Verification items for the finished model (mm, model axes). A direction names the side the tool comes from. Coordinates: 2 decimals unless noted, no trailing zeros. Loops run counter-clockwise (first coordinate to the right, second up) from the corner with the lowest first, then second, coordinate; pieces in that order, holes last. Notation, with made-up numbers: (12.5, -25) - (39.5, -25) arc R20 cw to (39.5, -1) - close; hole circle Ø10 at (-19.75, 0). An arc over 180 degrees is marked (long way). One line per item, written item: value. Start each with the question number.
(1) Set-up check for faces 4 (the face through (111, 69, 3)), 5 (the face through (64, 25, 28)): record each of +Z, -Z, +X, -X, +Y, -Y from which the full face is reachable in a straight line by a thin tool's end or side.
(2) Thickness scan on probe 1 along Y at (x, z) = (16.63, 16.25); probe 2 along Y at (x, z) = (49, 11.5); probe 3 along Y at (x, z) = (63.88, 14.25). Record the ranges inside material, lowest first. Write a range as [from, to].
(3) Draft check along X on faces 1 (the face through (92.562, 10.878, 13.919)), 2 (the face through (64, 4, 28)), 3 (the face through (0, 42, 14)). Enter one of: +X half, -X half, draft (parallel to the pull), parting line (faces both ways), or undercut.
(4) Gauge pin test, flat ends, axial feed: P1, Ø14, axis at x = 82.5, y = 14.5, coming from the +Z side; P2, Ø1.5, axis at x = 27, y = 56, coming from the +Z side; P3, Ø22.5, axis at x = 94, y = 46.5, coming from the +Z side. Record the tip position at first contact, or that the pin passes through.
(5) Section check A-A (z = 13.25). Count the separate pieces of the cut face and the enclosed holes in it, plus the area to 3 significant figures.
(6) Section check B-B (y = 42.74). Record the boundary of the cut face in (x, z), plus the area to 3 significant figures.
```python
from build123d import *

# Parameters (mm, degrees)
ESQUISSE1_W             = 127.76
ESQUISSE1_H             = 85.48
BOSS_EXTRU_1_DEPTH      = 28
ESQUISSE2_R             = 14
ENL_V_MAT_EXTRU_1_DEPTH = 25
CHANFREIN1_SIZE         = 2
CHANFREIN1_SIZE_2       = 3.464101615


with BuildPart() as part:
    # Esquisse1 → Boss.-Extru.1 (new body)
    with BuildSketch(Plane.XY):
        with Locations((63.88, 42.74)):
            Rectangle(ESQUISSE1_W, ESQUISSE1_H)
    extrude(amount=BOSS_EXTRU_1_DEPTH)

    # Esquisse2 → Enlèv. mat.-Extru.1 (cut)
    with BuildSketch(Plane.XY.offset(28)):
        with Locations((111.13, 69.24)):
            Circle(ESQUISSE2_R)
        with Locations((79.63, 69.24)):
            Circle(ESQUISSE2_R)
        with Locations((48.13, 69.24)):
            Circle(ESQUISSE2_R)
        with Locations((16.63, 69.24)):
            Circle(ESQUISSE2_R)
        with Locations((32.38, 42.74)):
            Circle(ESQUISSE2_R)
        with Locations((16.63, 16.24)):
            Circle(ESQUISSE2_R)
        with Locations((48.13, 16.24)):
            Circle(ESQUISSE2_R)
        with Locations((111.13, 16.24)):
            Circle(ESQUISSE2_R)
        with Locations((79.63, 16.24)):
            Circle(ESQUISSE2_R)
        with Locations((63.88, 42.74)):
            Circle(ESQUISSE2_R)
        with Locations((95.38, 42.74)):
            Circle(ESQUISSE2_R)
    extrude(amount=-ENL_V_MAT_EXTRU_1_DEPTH, mode=Mode.SUBTRACT)

    # Chanfrein1
    # the kernel refuses this chamfer: 3.464101615, 2 mm, written as the material it takes off along each edge
    with BuildSketch(Plane(origin=(79.63, 69.24, 28), x_dir=(1, 0, 0), z_dir=(0, -1, 0))) as chanfrein1_piece_1:
        Polygon((14 + CHANFREIN1_SIZE, 0), (14, -CHANFREIN1_SIZE_2), (14, 0), align=None)
    revolve(axis=Axis((79.63, 69.24, 28), (0, 0, 1)), mode=Mode.SUBTRACT)
    with BuildSketch(Plane(origin=(111.13, 69.24, 28), x_dir=(1, 0, 0), z_dir=(0, -1, 0))) as chanfrein1_piece_2:
        Polygon((14 + CHANFREIN1_SIZE, 0), (14, -CHANFREIN1_SIZE_2), (14, 0), align=None)
    revolve(axis=Axis((111.13, 69.24, 28), (0, 0, 1)), mode=Mode.SUBTRACT)
    with BuildSketch(Plane(origin=(63.88, 42.74, 28), x_dir=(1, 0, 0), z_dir=(0, -1, 0))) as chanfrein1_piece_3:
        Polygon((14 + CHANFREIN1_SIZE, 0), (14, -CHANFREIN1_SIZE_2), (14, 0), align=None)
    revolve(axis=Axis((63.88, 42.74, 28), (0, 0, 1)), mode=Mode.SUBTRACT)
    with BuildSketch(Plane(origin=(95.38, 42.74, 28), x_dir=(1, 0, 0), z_dir=(0, -1, 0))) as chanfrein1_piece_4:
        Polygon((14 + CHANFREIN1_SIZE, 0), (14, -CHANFREIN1_SIZE_2), (14, 0), align=None)
    revolve(axis=Axis((95.38, 42.74, 28), (0, 0, 1)), mode=Mode.SUBTRACT)
    with BuildSketch(Plane(origin=(32.38, 42.74, 28), x_dir=(1, 0, 0), z_dir=(0, -1, 0))) as chanfrein1_piece_5:
        Polygon((14 + CHANFREIN1_SIZE, 0), (14, -CHANFREIN1_SIZE_2), (14, 0), align=None)
    revolve(axis=Axis((32.38, 42.74, 28), (0, 0, 1)), mode=Mode.SUBTRACT)
    with BuildSketch(Plane(origin=(16.63, 16.24, 28), x_dir=(1, 0, 0), z_dir=(0, -1, 0))) as chanfrein1_piece_6:
        Polygon((14 + CHANFREIN1_SIZE, 0), (14, -CHANFREIN1_SIZE_2), (14, 0), align=None)
    revolve(axis=Axis((16.63, 16.24, 28), (0, 0, 1)), mode=Mode.SUBTRACT)
    with BuildSketch(Plane(origin=(16.63, 69.24, 28), x_dir=(1, 0, 0), z_dir=(0, -1, 0))) as chanfrein1_piece_7:
        Polygon((14 + CHANFREIN1_SIZE, 0), (14, -CHANFREIN1_SIZE_2), (14, 0), align=None)
    revolve(axis=Axis((16.63, 69.24, 28), (0, 0, 1)), mode=Mode.SUBTRACT)
    with BuildSketch(Plane(origin=(48.13, 69.24, 28), x_dir=(1, 0, 0), z_dir=(0, -1, 0))) as chanfrein1_piece_8:
        Polygon((14 + CHANFREIN1_SIZE, 0), (14, -CHANFREIN1_SIZE_2), (14, 0), align=None)
    revolve(axis=Axis((48.13, 69.24, 28), (0, 0, 1)), mode=Mode.SUBTRACT)
    with BuildSketch(Plane(origin=(79.63, 16.24, 28), x_dir=(1, 0, 0), z_dir=(0, -1, 0))) as chanfrein1_piece_9:
        Polygon((14 + CHANFREIN1_SIZE, 0), (14, -CHANFREIN1_SIZE_2), (14, 0), align=None)
    revolve(axis=Axis((79.63, 16.24, 28), (0, 0, 1)), mode=Mode.SUBTRACT)
    with BuildSketch(Plane(origin=(111.13, 16.24, 28), x_dir=(1, 0, 0), z_dir=(0, -1, 0))) as chanfrein1_piece_10:
        Polygon((14 + CHANFREIN1_SIZE, 0), (14, -CHANFREIN1_SIZE_2), (14, 0), align=None)
    revolve(axis=Axis((111.13, 16.24, 28), (0, 0, 1)), mode=Mode.SUBTRACT)
    with BuildSketch(Plane(origin=(48.13, 16.24, 28), x_dir=(1, 0, 0), z_dir=(0, -1, 0))) as chanfrein1_piece_11:
        Polygon((14 + CHANFREIN1_SIZE, 0), (14, -CHANFREIN1_SIZE_2), (14, 0), align=None)
    revolve(axis=Axis((48.13, 16.24, 28), (0, 0, 1)), mode=Mode.SUBTRACT)

    # Chanfrein2
    # the kernel refuses this chamfer: 1 mm, written as the material it takes off along each edge
    with BuildSketch(Plane(origin=(127.093333333, 0.666666667, 27.333333333), x_dir=(0.7071067811865476, 0.7071067811865474, 0), z_dir=(0.5773502691896257, -0.5773502691896258, 0.5773502691896258)), Plane(origin=(0.666666667, 84.813333333, 27.333333333), x_dir=(0.7071067811865475, 0, 0.7071067811865476), z_dir=(-0.5773502691896258, 0.5773502691896256, 0.5773502691896257)), Plane(origin=(127.093333333, 84.813333333, 0.666666667), x_dir=(-0.7071067811865476, 0, -0.7071067811865474), z_dir=(0.5773502691896257, 0.5773502691896257, -0.5773502691896258)), Plane(origin=(0.666666667, 0.666666667, 0.666666667), x_dir=(-0.7071067811865475, 0.7071067811865475, 0), z_dir=(-0.5773502691896257, -0.5773502691896257, -0.5773502691896257))) as chanfrein2_piece_1:
        Polygon((-0.707106781, -0.40824829), (0.707106781, -0.40824829), (0, 0.816496581), align=None)
    extrude(amount=1.270170592, mode=Mode.SUBTRACT)
    with BuildSketch(Plane(origin=(127.093333333, 84.813333333, 27.333333333), x_dir=(-0.7071067811865475, 0, 0.7071067811865475), z_dir=(0.5773502691896258, 0.5773502691896258, 0.5773502691896258)), Plane(origin=(0.666666667, 0.666666667, 27.333333333), x_dir=(-0.7071067811865475, 0.7071067811865475, 0), z_dir=(-0.5773502691896258, -0.5773502691896258, 0.5773502691896257)), Plane(origin=(0.666666667, 84.813333333, 0.666666667), x_dir=(0.7071067811865475, 0, -0.7071067811865475), z_dir=(-0.5773502691896258, 0.5773502691896256, -0.5773502691896258)), Plane(origin=(127.093333333, 0.666666667, 0.666666667), x_dir=(0.7071067811865476, 0.7071067811865475, 0), z_dir=(0.5773502691896256, -0.5773502691896258, -0.577350269189626))) as chanfrein2_piece_2:
        Polygon((-0.707106781, 0.40824829), (0.707106781, 0.40824829), (0, -0.816496581), align=None)
    extrude(amount=1.270170592, mode=Mode.SUBTRACT)
    with BuildSketch(Plane(origin=(127.76, -2.571682988, 28), x_dir=(0.0274958766105822, 0, -0.999621916911297), z_dir=(0, 1, 0)), Plane(origin=(0, 88.051682988, 28), x_dir=(-0.02749587661058639, 0, -0.9996219169112968), z_dir=(0, -1, 0))) as chanfrein2_piece_3:
        with BuildLine():
            Line((1.028673195, 0), (-0.056547155, 1.027117794))
            Line((-0.056547155, 1.027117794), (-0.076539593, 1.026567876))
            ThreePointArc((-0.076539593, 1.026567876), (-0.034129227, 0.51339783), (-0.019992438, -0.000549918))
            Line((-0.019992438, -0.000549918), (0.000549918, -0.019992438))
            ThreePointArc((0.000549918, -0.019992438), (0.514497665, -0.00585565), (1.029223113, -0.019992438))
            Line((1.029223113, -0.019992438), (1.028673195, 0))
        make_face()
    extrude(amount=90.623365976, mode=Mode.SUBTRACT)
    with BuildSketch(Plane(origin=(130.331682988, 85.48, 28), x_dir=(0, -0.9996219169112968, 0.02749587661058574), z_dir=(-1, 0, 0)), Plane(origin=(-2.571682988, 0, 0), x_dir=(0, -0.027495876610586372, 0.9996219169112968), z_dir=(1, 0, 0))) as chanfrein2_piece_4:
        with BuildLine():
            Line((1.028673195, 0), (-0.056547155, -1.027117794))
            Line((-0.056547155, -1.027117794), (-0.076539593, -1.026567876))
            ThreePointArc((-0.076539593, -1.026567876), (-0.034129227, -0.51339783), (-0.019992438, 0.000549918))
            Line((-0.019992438, 0.000549918), (0.000549918, 0.019992438))
            ThreePointArc((0.000549918, 0.019992438), (0.514497665, 0.00585565), (1.029223113, 0.019992438))
            Line((1.029223113, 0.019992438), (1.028673195, 0))
        make_face()
    extrude(amount=132.903365976, mode=Mode.SUBTRACT)
    with BuildSketch(Plane(origin=(130.331682988, 85.48, 0), x_dir=(0, -0.9996219169112968, -0.027495876610586483), z_dir=(-1, 0, 0)), Plane(origin=(-2.571682988, 0, 28), x_dir=(0, -0.02749587661058639, -0.9996219169112968), z_dir=(1, 0, 0))) as chanfrein2_piece_5:
        with BuildLine():
            Line((1.028673195, 0), (-0.056547155, 1.027117794))
            Line((-0.056547155, 1.027117794), (-0.076539593, 1.026567876))
            ThreePointArc((-0.076539593, 1.026567876), (-0.034129227, 0.51339783), (-0.019992438, -0.000549918))
            Line((-0.019992438, -0.000549918), (0.000549918, -0.019992438))
            ThreePointArc((0.000549918, -0.019992438), (0.514497665, -0.00585565), (1.029223113, -0.019992438))
            Line((1.029223113, -0.019992438), (1.028673195, 0))
        make_face()
    extrude(amount=132.903365976, mode=Mode.SUBTRACT)
    with BuildSketch(Plane(origin=(127.76, -2.571682988, 0), x_dir=(0.027495876610582174, 0, 0.9996219169112968), z_dir=(0, 1, 0)), Plane(origin=(0, 88.051682988, 0), x_dir=(-0.027495876610586372, 0, 0.9996219169112968), z_dir=(0, -1, 0))) as chanfrein2_piece_6:
        with BuildLine():
            Line((1.028673195, 0), (-0.056547155, -1.027117794))
            Line((-0.056547155, -1.027117794), (-0.076539593, -1.026567876))
            ThreePointArc((-0.076539593, -1.026567876), (-0.034129227, -0.51339783), (-0.019992438, 0.000549918))
            Line((-0.019992438, 0.000549918), (0.000549918, 0.019992438))
            ThreePointArc((0.000549918, 0.019992438), (0.514497665, 0.00585565), (1.029223113, 0.019992438))
            Line((1.029223113, 0.019992438), (1.028673195, 0))
        make_face()
    extrude(amount=90.623365976, mode=Mode.SUBTRACT)
    with BuildSketch(Plane(origin=(0, 85.48, -2.571682988), x_dir=(-0.027495876610586483, -0.9996219169112968, 0), z_dir=(0, 0, 1)), Plane(origin=(0, 0, -2.571682988), x_dir=(0.9996219169112968, -0.027495876610586372, 0), z_dir=(0, 0, 1))) as chanfrein2_piece_7:
        with BuildLine():
            Line((1.028673195, 0), (-0.056547155, 1.027117794))
            Line((-0.056547155, 1.027117794), (-0.076539593, 1.026567876))
            ThreePointArc((-0.076539593, 1.026567876), (-0.034129227, 0.51339783), (-0.019992438, -0.000549918))
            Line((-0.019992438, -0.000549918), (0.000549918, -0.019992438))
            ThreePointArc((0.000549918, -0.019992438), (0.514497665, -0.00585565), (1.029223113, -0.019992438))
            Line((1.029223113, -0.019992438), (1.028673195, 0))
        make_face()
    extrude(amount=33.143365976, mode=Mode.SUBTRACT)
    with BuildSketch(Plane(origin=(127.76, 85.48, -2.571682988), x_dir=(0.02749587661058229, -0.9996219169112968, 0), z_dir=(0, 0, 1)), Plane(origin=(127.76, 0, -2.571682988), x_dir=(-0.9996219169112968, -0.027495876610586483, 0), z_dir=(0, 0, 1))) as chanfrein2_piece_8:
        with BuildLine():
            Line((1.028673195, 0), (-0.056547155, -1.027117794))
            Line((-0.056547155, -1.027117794), (-0.076539593, -1.026567876))
            ThreePointArc((-0.076539593, -1.026567876), (-0.034129227, -0.51339783), (-0.019992438, 0.000549918))
            Line((-0.019992438, 0.000549918), (0.000549918, 0.019992438))
            ThreePointArc((0.000549918, 0.019992438), (0.514497665, 0.00585565), (1.029223113, 0.019992438))
            Line((1.029223113, 0.019992438), (1.028673195, 0))
        make_face()
    extrude(amount=33.143365976, mode=Mode.SUBTRACT)


solid = part.part
```
Responses:
1. face 4: +Z
1. face 5: +Z, +X, -X, +Y, -Y
2. probe 1: y = [0, 2.24], [30.24, 55.24], [83.24, 85.48]
2. probe 2: y = [0, 2.27], [30.21, 55.27], [83.21, 85.48]
2. probe 3: y = [0, 28.74], [56.74, 85.48]
3. face 1: undercut
3. face 2: draft
3. face 3: -X half
4. P1: stops at z = 3
4. P2: stops at z = 26.37
4. P3: stops at z = 26.71
5. separate pieces: 1
5. enclosed holes: 11
5. area: 4,150 mm²
6. outline: (0, 1) - (1, 0) - (126.76, 0) - (127.76, 1) - (127.76, 27) - (126.76, 28) - (111.38, 28) - (109.38, 24.54) - (109.38, 3) - (81.38, 3) - (81.38, 24.54) - (79.63, 27.57) - (77.88, 24.54) - (77.88, 3) - (49.88, 3) - (49.88, 24.54) - (48.13, 27.57) - (46.38, 24.54) - (46.38, 3) - (18.38, 3) - (18.38, 24.54) - (16.38, 28) - (1, 28) - (0, 27) - close
6. area: 1,450 mm²
